The listing builds one solid part. Answer for the finished solid, in the listing's coordinates (mm). Face numbers are marked on the shaded views. Give positions to 0.01 mm unless a question says otherwise; leave off trailing zeros. Loops run counter-clockwise (first coordinate to the right, second up) from the corner with the lowest first, then second, coordinate; pieces in that order, holes last. Notation, with made-up numbers: M 51.5,-2 L 106.5,-2 A18 ccw 106.5,11 Z; hole C 83.5,-39.5 d2. An arc over 180 degrees is marked long. Use one line per item in the form item = value. Start each with the question number.
1. The part is cut by section A-A (z = 1.5). Write down the section's boundary in (x, y) (3 decimals).
2. Straight lines are drawn through the part: line 1 (Y direction, x = -75, z = 5.05); line 2 (Y direction, x = 75, z = 2); line 3 (X direction, y = -4, z = 4.75). For each, find the intervals that lie inside material, in ascending order. Write a range as from..to.
3. The part is cut by section C-C (x = -17.5). Write down the section's boundary in (y, z), and give its area (3 significant figures).
4. Each of these flat-tipped pins is pushed along its axis until it touches: pin 1 Ø1.9 at (x, y) = (75, 0) entering from -Z; pin 2 Ø1 at (y, z) = (4.5, 1) entering from +X; pin 3 Ø6 at (x, y) = (19, 2.5) entering from +Z; pin 4 Ø5 at (x, y) = (71.5, -4) entering from +Z. Where does it stop, or does it pass through?
5. The mould has two halves that part along Y. Classify the marked faces 1 and 2: released by +Y, released by -Y, zero draft, split by the parting line, or undercut.
6. The part is cut by section B-B (y = 0). Give the number of separate pieces and of enclosed holes in the cut face, and give its area (3 significant figures).
from build123d import *

# Parameters (mm, degrees)
BASE_R              = 2.6
BASE_R_2            = 8.1
BASE_R_3            = 1.55
BOSS_EXTRUDE1_DEPTH = 4
BOSS_EXTRUDE2_START = 4
BASE_3_R            = 8.1
BASE_3_R_2          = 2.6
BASE_3_R_3          = 1.55
BOSS_EXTRUDE2_DEPTH = 2.5
SKETCH2_R           = 3
CUT_EXTRUDE1_DEPTH  = 3
CUT_EXTRUDE2_DEPTH  = 2
FILLET1_R           = 0.5


with BuildPart() as part:
    # Base → Boss-Extrude1 (new body)
    with BuildSketch(Plane.XY):
        with BuildLine():
            ThreePointArc((75, 10), (85, 0), (75, -10))
            Line((75, -10), (-75, -10))
            ThreePointArc((-75, -10), (-85, 0), (-75, 10))
            Line((-75, 10), (75, 10))
        make_face()
        with Locations((75, 0)):
            Circle(BASE_R, mode=Mode.SUBTRACT)
        with Locations((-75, 0)):
            Circle(BASE_R, mode=Mode.SUBTRACT)
        with Locations((75, 0)):
            Circle(BASE_R_2)
        with Locations((75, 0)):
            Circle(BASE_R, mode=Mode.SUBTRACT)
        with Locations((75, 0)):
            Circle(BASE_R)
        with Locations((75, 0)):
            Circle(BASE_R_3, mode=Mode.SUBTRACT)
        with Locations((-75, 0)):
            Circle(BASE_R_2)
        with Locations((-75, 0)):
            Circle(BASE_R, mode=Mode.SUBTRACT)
        with Locations((-75, 0)):
            Circle(BASE_R)
        with Locations((-75, 0)):
            Circle(BASE_R_3, mode=Mode.SUBTRACT)
    extrude(amount=BOSS_EXTRUDE1_DEPTH)

    # Base<3> → Boss-Extrude2 (add)
    with BuildSketch(Plane.XY.offset(BOSS_EXTRUDE2_START)):
        with BuildLine():
            ThreePointArc((75, 10), (85, 0), (75, -10))
            Line((75, -10), (-75, -10))
            ThreePointArc((-75, -10), (-85, 0), (-75, 10))
            Line((-75, 10), (75, 10))
        make_face()
        with Locations((-75, 0)):
            Circle(BASE_3_R, mode=Mode.SUBTRACT)
        with Locations((75, 0)):
            Circle(BASE_3_R, mode=Mode.SUBTRACT)
        with Locations((75, 0)):
            Circle(BASE_3_R_2)
        with Locations((75, 0)):
            Circle(BASE_3_R_3, mode=Mode.SUBTRACT)
        with Locations((-75, 0)):
            Circle(BASE_3_R_2)
        with Locations((-75, 0)):
            Circle(BASE_3_R_3, mode=Mode.SUBTRACT)
    extrude(amount=BOSS_EXTRUDE2_DEPTH)

    # Sketch2 → Cut-Extrude1 (cut)
    with BuildSketch(Plane(origin=(0, 0, 0), x_dir=(-1, 0, 0), z_dir=(0, 0, -1))):
        with Locations((-75, 0)):
            Circle(SKETCH2_R)
        Polygon((72.125, 1.659882024), (72.125, -1.659882024), (75, -3.319764048), (77.875, -1.659882024), (77.875, 1.659882024), (75, 3.319764048), align=None)
    extrude(amount=-CUT_EXTRUDE1_DEPTH, mode=Mode.SUBTRACT)

    # Sketch3 → Cut-Extrude2 (cut)
    with BuildSketch(Plane.XY.offset(6.5)):
        with BuildLine():
            Line((66.385477378, -7), (-66.385477378, -7))
            ThreePointArc((-66.385477378, -7), (-63.9, 0), (-66.385477378, 7))
            Line((-66.385477378, 7), (66.385477378, 7))
            ThreePointArc((66.385477378, 7), (63.9, 0), (66.385477378, -7))
        make_face()
    extrude(amount=-CUT_EXTRUDE2_DEPTH, mode=Mode.SUBTRACT)

    # Fillet1
    fillet1_edges = [part.edges().sort_by_distance(p)[0] for p in [
        (85, 0, 6.5),
        (0, 10, 6.5),
        (-85, 0, 6.5),
        (0, -10, 6.5),
        (63.9, 0, 6.5),
        (0, 7, 6.5),
        (-63.9, 0, 6.5),
        (0, -7, 6.5),
    ]]
    fillet(fillet1_edges, radius=FILLET1_R)


solid = part.part
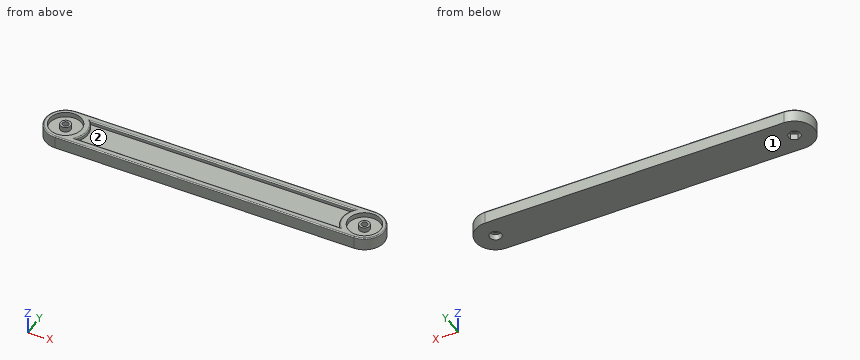
Derived:
q1.outline = M -75,-10 L 75,-10 A10 ccw 75,10 L -75,10 A10 ccw Z; hole M -77.875,-1.66 L -75,-3.32 L -72.125,-1.66 L -72.125,1.66 L -75,3.32 L -77.875,1.66 Z; hole C 75,0 d6
q2.line_1 = -10..-8.1, -2.6..-1.55, 1.55..2.6, 8.1..10
q2.line_2 = -10..-3, 3..10
q2.line_3 = -84.17..-82.04, -67.96..-64.65, 64.65..67.96, 82.04..84.17
q3.outline = M -10,0 L 10,0 L 10,6 A0.5 ccw 9.5,6.5 L 7.5,6.5 A0.5 ccw 7,6 L 7,4.5 L -7,4.5 L -7,6 A0.5 ccw -7.5,6.5 L -9.5,6.5 A0.5 ccw -10,6 Z
q3.area = 102 mm2
q4.pin_1 = through
q4.pin_2 = 84.17
q4.pin_3 = 4.5
q4.pin_4 = 4
q5.face_1 = zero draft
q5.face_2 = undercut
q6.separate_pieces = 3
q6.enclosed_holes = 0
q6.area = 737 mm2
